Here's the drawing with two shaded views (mm, measured from the low corner). I have some questions. A direction names the side the tool comes from. Give positions to 0.01 mm unless a question says otherwise; leave off trailing zeros. Order: outer loops, then holes, each group sorted by start corner. A loop starts at its lowest first (then second) coordinate and runs counter-clockwise, first axis right, second up. Notation, with made-up numbers: (44, 64.5) - (51, 64.5) arc R10 ccw to (51, 73.5) - close; hole circle Ø4 at (-11.5, 80). An arc over 180 degrees is marked (long way). Use one line per item in the form item = value. Start each with the question number.
1) Suppose I cut it at A-A, the plane y = 31. Write out the boundary of the cut face in (x, z).
2) Please list where these lines run through material, in increasing order: probe 1 along Y at (x, z) = (31, 6.75); probe 2 along X at (y, z) = (16.5, 3.5); probe 3 along X at (y, z) = (36, 7.25).
3) Which directions (+Z, -Z, +X, -X, +Y, -Y) give clear straight access to the entire face, cutting with the end or side of a thin tool? Please do the marked faces 1 and 2.
4) We'd pull the mould along Y, two halves only. Please class the marked faces 3, 4 and 5: released by +Y, released by -Y, zero draft, split by the parting line, or undercut.
5) Suppose I cut it at D-D, the plane x = 5. Write out the boundary of the cut face in (y, z).
6) Suppose I cut it at C-C, the plane z = 6.25. Write out the boundary of the cut face in (x, y), and give its area (3 significant figures).
7) For pin 1 (2 mm diameter, centred on y = 26.5, z = 2, fed in from -X); pin 2 (2 mm diameter, centred on y = 55, z = 8, fed in from +X); pin 3 (2 mm diameter, centred on x = 42.5, y = 8, fed in from +Z), each with a flat end and sliding along its axis, tell me the tip position at first contact or that it passes through.
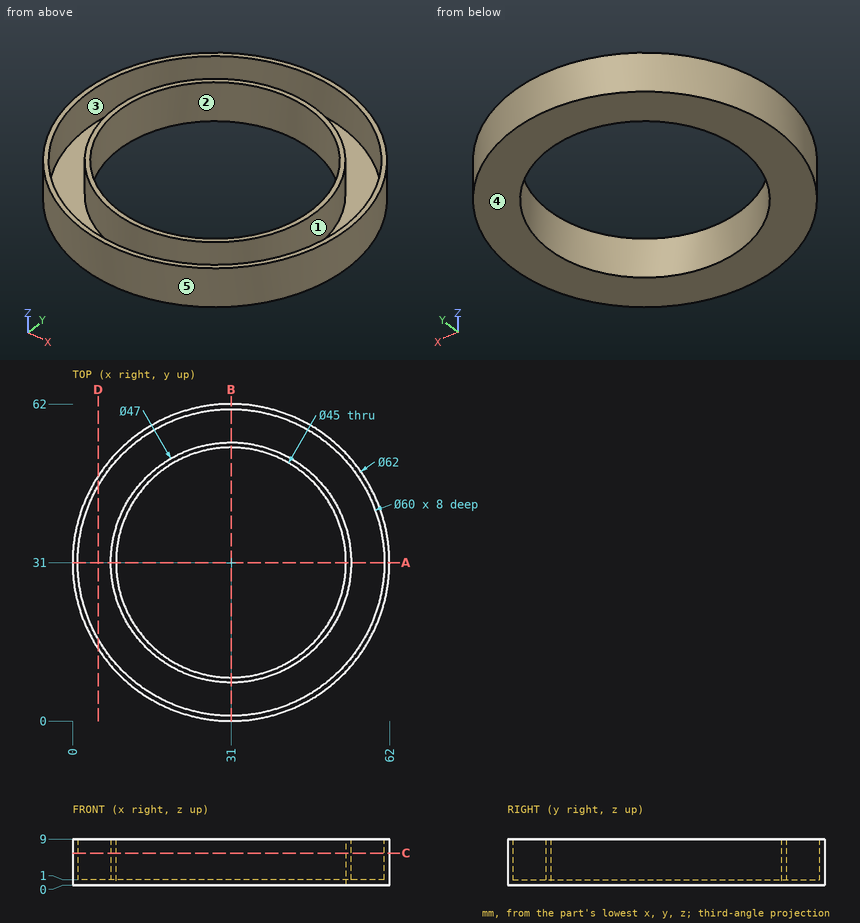
Result sheet:
q1.outline = (0, 0) - (8.5, 0) - (8.5, 9) - (7.5, 9) - (7.5, 1) - (1, 1) - (1, 9) - (0, 9) - close; (53.5, 0) - (62, 0) - (62, 9) - (61, 9) - (61, 1) - (54.5, 1) - (54.5, 9) - (53.5, 9) - close
q2.probe_1 = 0 to 1, 7.5 to 8.5, 53.5 to 54.5, 61 to 62
q2.probe_2 = 3.6 to 4.74, 12.51 to 13.8, 48.2 to 49.49, 57.26 to 58.4
q2.probe_3 = 0.41 to 1.42, 8.04 to 9.06, 52.94 to 53.96, 60.58 to 61.59
q3.face_1 = +Z
q3.face_2 = +Z, -Z
q4.face_3 = undercut
q4.face_4 = zero draft
q4.face_5 = split by the parting line
q5.outline = (14.12, 0) - (47.88, 0) - (47.88, 9) - (45.97, 9) - (45.97, 1) - (16.03, 1) - (16.03, 9) - (14.12, 9) - close
q6.outline = circle Ø62 at (31, 31); circle Ø47 at (31, 31); hole circle Ø60 at (31, 31); hole circle Ø45 at (31, 31)
q6.area = 336 mm²
q7.pin_1 = 0.2
q7.pin_2 = 51.78
q7.pin_3 = 1
